Part model, mm, in its own coordinate system. Round coordinates to 2 decimals unless told otherwise and drop trailing zeros. Write each loop counter-clockwise with the first axis right and the second up, starting at its lowest first coordinate (ties: lowest second). Pieces come first, ordered by that corner, then holes.
```python
from build123d import *

# Parameters (mm, degrees)
SKETCH1_W                = 350
SKETCH1_H                = 200
BOSS_EXTRUDE1_DEPTH      = 5
M4_CLEARANCE_HOLE2_D     = 4.5
M4_CLEARANCE_HOLE2_DEPTH = 10
M4_CLEARANCE_HOLE2_TIP   = 1.351936393
SKETCH8_R                = 3
CUT_EXTRUDE2_DEPTH       = 404.143894906
SKETCH10_W               = 110
SKETCH10_H               = 200
CUT_EXTRUDE4_DEPTH       = 404.143894906
SKETCH11_W               = 240
SKETCH11_H               = 25
BOSS_EXTRUDE2_DEPTH      = 5
M8_CLEARANCE_HOLE1_D     = 9
FILLET3_R                = 5


with BuildPart() as part:
    # Sketch1 → Boss-Extrude1 (new body)
    with BuildSketch(Plane(origin=(0, 0, 0), x_dir=(1, 0, 0), z_dir=(0, 1, 0))):
        with Locations((175, 100)):
            Rectangle(SKETCH1_W, SKETCH1_H)
    extrude(amount=BOSS_EXTRUDE1_DEPTH)

    # M4 Clearance Hole2
    with Locations(Plane(origin=(0, 5, 0), x_dir=(1, 0, 0), z_dir=(0, 1, 0))):
        with Locations((279.726995352, 76.5), (279.726995352, 123.5), (303.226995352, 100), (256.226995352, 100)):
            Hole(M4_CLEARANCE_HOLE2_D / 2, depth=M4_CLEARANCE_HOLE2_DEPTH)
            with Locations((0, 0, -(M4_CLEARANCE_HOLE2_DEPTH + M4_CLEARANCE_HOLE2_TIP / 2))):  # 118° drill point
                Cone(0, M4_CLEARANCE_HOLE2_D / 2, M4_CLEARANCE_HOLE2_TIP, mode=Mode.SUBTRACT)

    # Sketch8 → Cut-Extrude2 (cut, through all)
    with BuildSketch(Plane(origin=(0, 5, 0), x_dir=(1, 0, 0), z_dir=(0, 1, 0))):
        with Locations(Location((159.999156247, 78, 0), (0, 0, 270))):
            Circle(SKETCH8_R)
        with BuildLine():
            Line((174.999156247, 81), (194.999156247, 81))
            ThreePointArc((194.999156247, 81), (197.999156247, 78), (194.999156247, 75))
            Line((194.999156247, 75), (174.999156247, 75))
            ThreePointArc((174.999156247, 75), (171.999156247, 78), (174.999156247, 81))
        make_face()
    extrude(amount=-CUT_EXTRUDE2_DEPTH, mode=Mode.SUBTRACT)

    # Sketch10 → Cut-Extrude4 (cut, through all)
    with BuildSketch(Plane(origin=(0, 5, 0), x_dir=(1, 0, 0), z_dir=(0, 1, 0))):
        with Locations((295, 100)):
            Rectangle(SKETCH10_W, SKETCH10_H)
    extrude(amount=-CUT_EXTRUDE4_DEPTH, mode=Mode.SUBTRACT)

    # Sketch11 → Boss-Extrude2 (add)
    with BuildSketch(Plane(origin=(0, 5, 0), x_dir=(1, 0, 0), z_dir=(0, 1, 0))):
        with Locations((120, 212.5)):
            Rectangle(SKETCH11_W, SKETCH11_H)
    extrude(amount=-BOSS_EXTRUDE2_DEPTH)

    # M8 Clearance Hole1 (through all)
    with Locations(Plane(origin=(0, 5, 0), x_dir=(1, 0, 0), z_dir=(0, 1, 0))):
        with Locations((15, 15), (225, 15), (225, 210), (15, 210)):
            Hole(M8_CLEARANCE_HOLE1_D / 2)

    # Fillet3
    fillet3_edges = [part.edges().sort_by_distance(p)[0] for p in [
        (240, 2.5, 0),
        (0, 2.5, 0),
        (0, 2.5, -225),
        (240, 2.5, -225),
    ]]
    fillet(fillet3_edges, radius=FILLET3_R)


solid = part.part
```
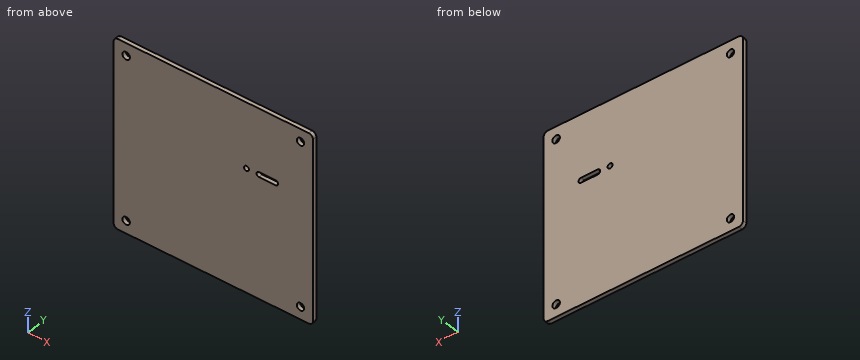
Q1. Cut at C-C on z = -15. Write the cut outline in (x, y).
Values follow:
outline: (0, 0) - (10.5, 0) - (10.5, 5) - (0, 5) - close; (19.5, 0) - (220.5, 0) - (220.5, 5) - (19.5, 5) - close; (229.5, 0) - (240, 0) - (240, 5) - (229.5, 5) - close
Q2. Cut at A-A on x = 225. Write the cut outline in (y, z), plus the area to 4 significant figures.
Values follow:
outline: (0, -225) - (5, -225) - (5, -214.5) - (0, -214.5) - close; (0, -205.5) - (5, -205.5) - (5, -19.5) - (0, -19.5) - close; (0, -10.5) - (5, -10.5) - (5, 0) - (0, 0) - close
area: 1,035 mm2
Q3. Cut at B-B on x = 183.5. Write the cut outline in (y, z).
Values follow:
outline: (0, -225) - (5, -225) - (5, -81) - (0, -81) - close; (0, -75) - (5, -75) - (5, 0) - (0, 0) - close
Q4. Wall check: L1, parallel to Z at x = 225, y = 2.35; L2, parallel to X at y = 2.35, z = -210; L3, parallel to X at y = 1.35, z = -78. Give the ranges that are in metal, low to high.
Values follow:
L1: z = -225 to -214.5, -205.5 to -19.5, -10.5 to 0
L2: x = 0 to 10.5, 19.5 to 220.5, 229.5 to 240
L3: x = 0 to 157, 163 to 172, 198 to 240
